Answer from the drawing. Dimensions are ordinates in mm from the lowest x, y and z of the part. A direction names the side the tool comes from. Round coordinates to 2 decimals unless told otherwise and drop trailing zeros. Loops run counter-clockwise (first coordinate to the right, second up) from the corner with the lowest first, then second, coordinate; pieces in that order, holes last. Notation, with made-up numbers: M 29.25,36.25 L 67.25,36.25 A21 cw 67.25,70.25 Z; hole C 46.5,-19.75 d1. An arc over 180 degrees is marked long. Write each question's results on one line, items separated by ' | '.
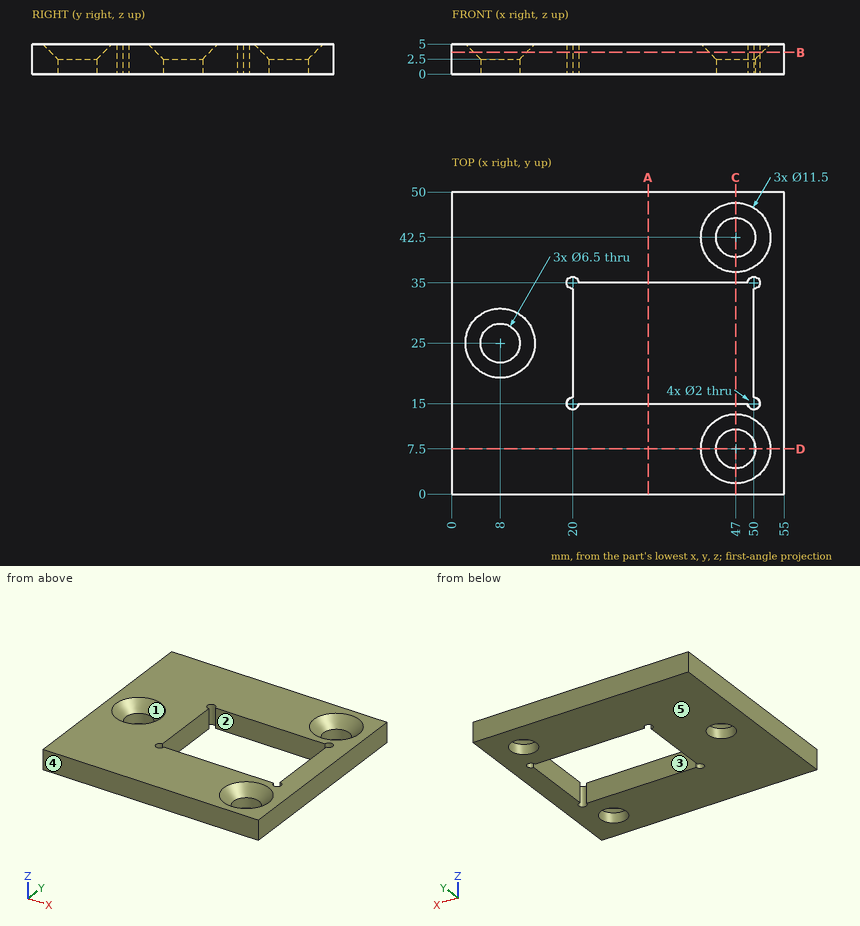
1. Find section D-D, the plane y = 7.5. Give the vertices of the cut face in (x, z), then the cut area to 3 significant figures.
Completed:
outline: M 0,0 L 43.75,0 L 43.75,2.5 L 41.25,5 L 0,5 Z; M 50.25,0 L 55,0 L 55,5 L 52.75,5 L 50.25,2.5 Z | area: 236 mm2
2. Find section B-B, the plane z = 3.6. Give the vertices of the cut face in (x, y), then the cut area to 3 significant figures.
Completed:
outline: M 0,0 L 55,0 L 55,50 L 0,50 Z; hole C 8,25 d8.7; hole M 20,16 A1 ccw long 21,15 L 49,15 A1 ccw long 50,16 L 50,34 A1 ccw long 49,35 L 21,35 A1 ccw long 20,34 Z; hole C 47,7.5 d8.7; hole C 47,42.5 d8.7 | area: 1,960 mm2
3. Find section C-C, the plane x = 47. Give the vertices of the cut face in (y, z).
Completed:
outline: M 0,0 L 4.25,0 L 4.25,2.5 L 1.75,5 L 0,5 Z; M 10.75,0 L 15,0 L 15,5 L 13.25,5 L 10.75,2.5 Z; M 35,0 L 39.25,0 L 39.25,2.5 L 36.75,5 L 35,5 Z; M 45.75,0 L 50,0 L 50,5 L 48.25,5 L 45.75,2.5 Z
4. Find section A-A, the plane x = 32.5. Give the vertices of the cut face in (y, z), then the cut area to 3 significant figures.
Completed:
outline: M 0,0 L 15,0 L 15,5 L 0,5 Z; M 35,0 L 50,0 L 50,5 L 35,5 Z | area: 150 mm2
5. Given P1, Ø1.5, axis at x = 29.5, y = 7, coming from the -Z side; P2, Ø7.5, axis at x = 47, y = 42.5, coming from the +Z side; P3, Ø1.5, axis at x = 44, y = 44, coming from the +Z side; P4, Ø5, axis at x = 47, y = 7.5, coming from the -Z side, each flat-ended and moving along its own axis, determine where each tip first touches the part or whether it passes through.
Completed:
P1: stops at z = 0 | P2: stops at z = 3 | P3: stops at z = 3.35 | P4: passes through
6. Find the intervals of material crossed by L1, parallel to X at y = 25, z = 1.9; L2, parallel to Y at x = 47, z = 1.9; L3, parallel to Y at x = 31.5, z = 4.6, in increasing order.
Completed:
L1: x = 0 to 4.75, 11.25 to 20, 50 to 55 | L2: y = 0 to 4.25, 10.75 to 15, 35 to 39.25, 45.75 to 50 | L3: y = 0 to 15, 35 to 50
7. Which of the six approach directions +Z, -Z, +X, -X, +Y, -Y give full straight-line access (tool end or side, diameter ignored) to the marked faces 1 and 2?
Completed:
face 1: +Z | face 2: +Z, -Z
8. Determine the mould class of the marked faces 3, 4 and 5 for opening direction Y: released by +Y, released by -Y, zero draft, split by the parting line, or undercut.
Completed:
face 3: undercut | face 4: released by -Y | face 5: zero draft
